For this review, take the finished solid that the model builds, in its own axes (mm). Give positions to 0.01 mm unless a question says otherwise; leave off trailing zeros. Order: outer loops, then holes, each group sorted by start corner. A loop starts at its lowest first (then second) coordinate and runs counter-clockwise, first axis right, second up.
Item 1: For probe 1 along X at (y, z) = (50, 0.25); probe 2 along Z at (x, y) = (-3.5, 41.5), list the stretches that pass through material, from the lowest coordinate up.
Item 2: Consider section A-A (y = 49). Give the boundary of the cut face in (x, z) (3 decimals).
Item 3: For P1, Ø0.8, axis at x = 3.5, y = 37, coming from the -Z side; P2, Ø0.6, axis at x = -3.5, y = 32.5, coming from the +Z side; P3, Ø0.6, axis at y = 14.5, z = 3.5, coming from the +X side, all flat-tipped, find the tip position at first contact; note any pin that passes through.
```python
from build123d import *

# Parameters (mm, degrees)
SKETCH1_R           = 3.875
BOSS_EXTRUDE1_DEPTH = 55
FILLET1_R           = 2
SKETCH2_W           = 2.5
SKETCH2_H           = 2.5
CUT_EXTRUDE1_DEPTH  = 56.272337121
CIRPATTERN1_COUNT   = 4
FILLET2_R           = 1.5


with BuildPart() as part:
    # Sketch1 → Boss-Extrude1 (new body)
    with BuildSketch(Plane(origin=(0, 0, 0), x_dir=(1, 0, 0), z_dir=(0, 1, 0))):
        with Locations(Location((0, 0, 0), (0, 0, 270))):
            Circle(SKETCH1_R)
    extrude(amount=BOSS_EXTRUDE1_DEPTH)

    # Fillet1
    fillet1_edges = [part.edges().sort_by_distance(p)[0] for p in [
        (0, 55, -3.875),
    ]]
    fillet(fillet1_edges, radius=FILLET1_R)

    # Sketch2 → Cut-Extrude1 (cut, through all)
    with BuildSketch(Plane(origin=(0, 55, 0), x_dir=(1, 0, 0), z_dir=(0, 1, 0))):
        with Locations((2.628858223, -2.628858223)):
            Rectangle(SKETCH2_W, SKETCH2_H)
    cut_extrude1 = extrude(amount=-CUT_EXTRUDE1_DEPTH, mode=Mode.SUBTRACT)

    # CirPattern1: Cut-Extrude1 ×4 about axis
    cirpattern1_axis = Axis((0, 0, 0), (0, 1, 0))
    for i in range(1, CIRPATTERN1_COUNT):
        add(cut_extrude1.rotate(cirpattern1_axis, i * 360 / CIRPATTERN1_COUNT), mode=Mode.SUBTRACT)

    # Fillet2
    fillet2_edges = [part.edges().sort_by_distance(p)[0] for p in [
        (1.378858223, 27.499296628, -1.378858223),
        (-1.378858223, 27.499296628, -1.378858223),
        (-1.378858223, 27.499296628, 1.378858223),
        (1.378858223, 27.499296628, 1.378858223),
    ]]
    fillet(fillet2_edges, radius=FILLET2_R)


solid = part.part
```
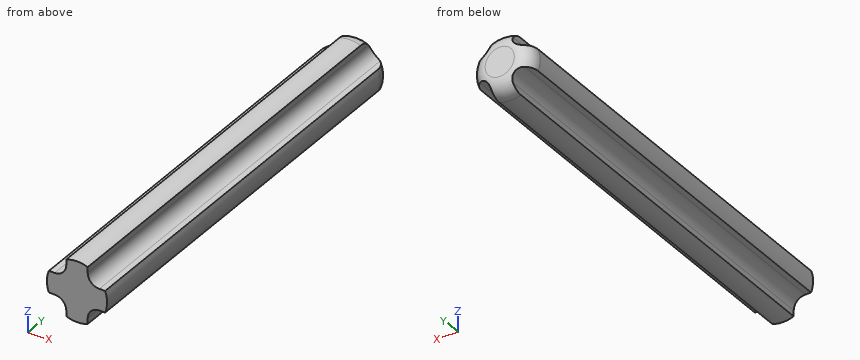
Resolved:
1. probe 1: x = -3.87 to 3.87
1. probe 2: z = -1.38 to 1.38
2. outline: (-3.621, -1.379) - (-2.879, -1.379) arc R1.5 cw to (-1.379, -2.879) - (-1.379, -3.621) arc R3.875 ccw to (1.379, -3.621) - (1.379, -2.879) arc R1.5 cw to (2.879, -1.379) - (3.621, -1.379) arc R3.875 ccw to (3.621, 1.379) - (2.879, 1.379) arc R1.5 cw to (1.379, 2.879) - (1.379, 3.621) arc R3.875 ccw to (-1.379, 3.621) - (-1.379, 2.879) arc R1.5 cw to (-2.879, 1.379) - (-3.621, 1.379) arc R3.875 ccw to start
3. P1: stops at z = -1.38
3. P2: stops at z = 1.38
3. P3: stops at x = 1.38
